Read the model definition and answer for the solid it produces. Units are mm, in the model's axes. A direction names the side the tool comes from. Give positions to 0.01 mm unless a question says otherwise; leave off trailing zeros. Order: outer loops, then holes, each group sorted by start corner. A loop starts at its lowest first (then second) coordinate and runs counter-clockwise, first axis right, second up.
Autodesk Inventor part; units mm, degrees
ref_plane "YZ Plane" through (0, 0, 0) normal (1, 0, 0) x (0, 1, 0)
ref_plane "XZ Plane" through (0, 0, 0) normal (0, 1, 0) x (-1, 0, 0)
ref_plane "XY Plane" through (0, 0, 0) normal (0, 0, 1) x (1, 0, 0)
sketch "スケッチ1" plane through (0, 0, 0) normal (0, 0, 1) x (1, 0, 0)
  circle A0 centre (0, 0) radius 4
  dimension "d0" = 8
extrude "押し出し1" add sketch "スケッチ1" along normal blind 35
hole "穴1" at (0, 0, 0) direction (0, 0, 1) diameter 4 depth 8 tip angle 118
sketch "スケッチ2" plane through (0, 0, 35) normal (0, 0, 1) x (1, 0, 0)
  point P0 (0, 0)
  point P1 (0, 0)
hole "穴2" at (0, 0, 35) direction (0, 0, -1) diameter 4 depth 8 tip angle 118
properties part number "スペーサ　m4-l35" material "アルミニウム 2014-T4"
1) The part is cut by section C-C on x = 2.75. Determine the outline of the cut face in (y, z).
Final values:
outline: (-2.9, 0) - (2.9, 0) - (2.9, 35) - (-2.9, 35) - close
2) For a pull along Y with two mould halves and no side action, classify faces 4 (the face through (0.104, 0.331, 8.993)), 5 (the face through (-0.867, 3.905, 17.255)), 6 (the face through (-0.34, 0.08, 26.01)), 7 (the face through (-2, -1, 0)) as released by +Y, released by -Y, zero draft, split by the parting line, or undercut.
Final values:
face 4: undercut
face 5: split by the parting line
face 6: undercut
face 7: zero draft
3) Consider L1, parallel to Y at x = 0, z = 3.25; L2, parallel to Y at x = 0.75, z = 32; L3, parallel to Z at x = -0.5, y = 1.5. Determine where each line is inside the solid, lowest interval first.
Final values:
L1: y = -4 to -2, 2 to 4
L2: y = -3.93 to -1.85, 1.85 to 3.93
L3: z = 8.25 to 26.75
4) A tool of negligible diameter and unlimited length cuts with its end or side. For faces 1 (the face through (2, 0, 31)), 2 (the face through (2, 0, 4)), 3 (the face through (-2, -1, 35)), from which of +Z, -Z, +X, -X, +Y, -Y can it reach the whole face along a straight path? Write none if from no direction.
Final values:
face 1: +Z
face 2: -Z
face 3: +Z, +X, -X, +Y, -Y
5) The part is cut by section B-B on y = 2.5. Determine the outline of the cut face in (x, z).
Final values:
outline: (-3.12, 0) - (3.12, 0) - (3.12, 35) - (-3.12, 35) - close
6) Given pin 1 (1.5 mm diameter, centred on y = -1, z = 23.5, fed in from -X); pin 2 (1.5 mm diameter, centred on x = 0, y = 0, fed in from +Z); pin 3 (3 mm diameter, centred on y = -2, z = 11, fed in from +X), each flat-ended and moving along its own axis, determine where each tip first touches the part or whether it passes through.
Final values:
pin 1: stops at x = -3.99
pin 2: stops at z = 26.25
pin 3: stops at x = 3.97
7) The part is cut by section A-A on z = 29.5. Determine the outline of the cut face in (x, y).
Final values:
outline: circle Ø8 at (0, 0); hole circle Ø4 at (0, 0)
